```python
from build123d import *

# Parameters (mm, degrees)
SKETCH_1_R          = 30
SKETCH_1_R_2        = 4
EXTRUDE_1_DEPTH     = 20
SKETCH_2_R          = 25
CUT_EXTRUDE_1_DEPTH = 16
FILLET_1_R          = 5


with BuildPart() as part:
    # 草图1 → 凸台-拉伸1 (new body)
    with BuildSketch(Plane.XY):
        Circle(SKETCH_1_R)
        Circle(SKETCH_1_R_2, mode=Mode.SUBTRACT)
    extrude(amount=EXTRUDE_1_DEPTH)

    # 草图2 → 切除-拉伸1 (cut)
    with BuildSketch(Plane.XY.offset(20)):
        Circle(SKETCH_2_R)
    extrude(amount=-CUT_EXTRUDE_1_DEPTH, mode=Mode.SUBTRACT)

    # 圆角1
    fillet_1_edges = [part.edges().sort_by_distance(p)[0] for p in [
        (-30, 0, 0),
        (-30, 0, 20),
    ]]
    fillet(fillet_1_edges, radius=FILLET_1_R - 0.0001)  # a hair under: the kernel refuses the full size


solid = part.part
```
Part model, mm, in its own coordinate system. A direction names the side the tool comes from. Round coordinates to 2 decimals unless told otherwise and drop trailing zeros. Write each loop counter-clockwise with the first axis right and the second up, starting at its lowest first coordinate (ties: lowest second). Pieces come first, ordered by that corner, then holes. Notation, with made-up numbers: (-2, -26) -> (53, -26) arc R15 cw to (53, 2) -> close; hole circle Ø1 at (-31, 23). An arc over 180 degrees is marked (long way). Return JSON: item names as keys, results as strings. Group by question number.
Q1. Which spindle directions (+Z, -Z, +X, -X, +Y, -Y) get a long thin tool onto all of the face, cutting with end or side? Do faces 4 (the flat face through (0, -5, 4)), 5 (the cylindrical face through (-0.867, -3.905, 1.972)). Say none if no direction does.
Q2. Pin check, flat tips, straight feed: pin 1 (1.5 mm diameter, centred on x = 20.5, z = 3.5, fed in from +Y); pin 2 (5 mm diameter, centred on x = -8.5, z = 2, fed in from +Y); pin 3 (12 mm diameter, centred on x = -9, z = 12.5, fed in from -Y). Stop position of each tip, or through.
Q3. Probe L1, parallel to Y at x = 0, z = 12.5; L2, parallel to Z at x = -15, y = 6.5; L3, parallel to Y at x = -3.5, z = 4.5. List the from-to ranges inside material, lowest first. Write a range as [from, to].
Q4. Saw through at C-C on z = 7. Write the cut outline in (x, y).
Q5. Mould opens along X. For faces 1 (the flat face through (0, -5, 0)), 2 (the cylindrical face through (23.846, 7.509, 12.112)), 3 (the cylindrical face through (-29.97, 1.32, 9.93)) say: pulls with the +X half, pulls with the -X half, needs draft (parallel to the pull), parting line crosses it, or undercut.
Answer:
{
 "1": {"face 4": "+Z", "face 5": "+Z, -Z"},
 "2": {"pin 1": "y = 22.33", "pin 2": "y = 29.08", "pin 3": "y = -29.85"},
 "3": {"L1": "[-30, -25], [25, 30]", "L2": "[0, 4]", "L3": "[-29.77, -24.75], [24.75, 29.77]"},
 "4": {"outline": "circle Ø60 at (0, 0); hole circle Ø50 at (0, 0)"},
 "5": {"face 1": "needs draft", "face 2": "undercut", "face 3": "parting line crosses it"}
}
